For this review, use the dimensioned drawing (mm, ordinates from the lowest corner) and the shaded views. Give positions to 0.01 mm unless a question says otherwise; leave off trailing zeros. Write each loop counter-clockwise with the first axis right and the second up, starting at its lowest first coordinate (ties: lowest second). Pieces come first, ordered by that corner, then holes. Notation, with made-up numbers: (-34, 7.5) -> (-9, 7.5) arc R26 cw to (-9, 42.5) -> close; hole circle Ø4 at (5.25, -9). An arc over 180 degrees is marked (long way). Answer as CSV lines item,"result".
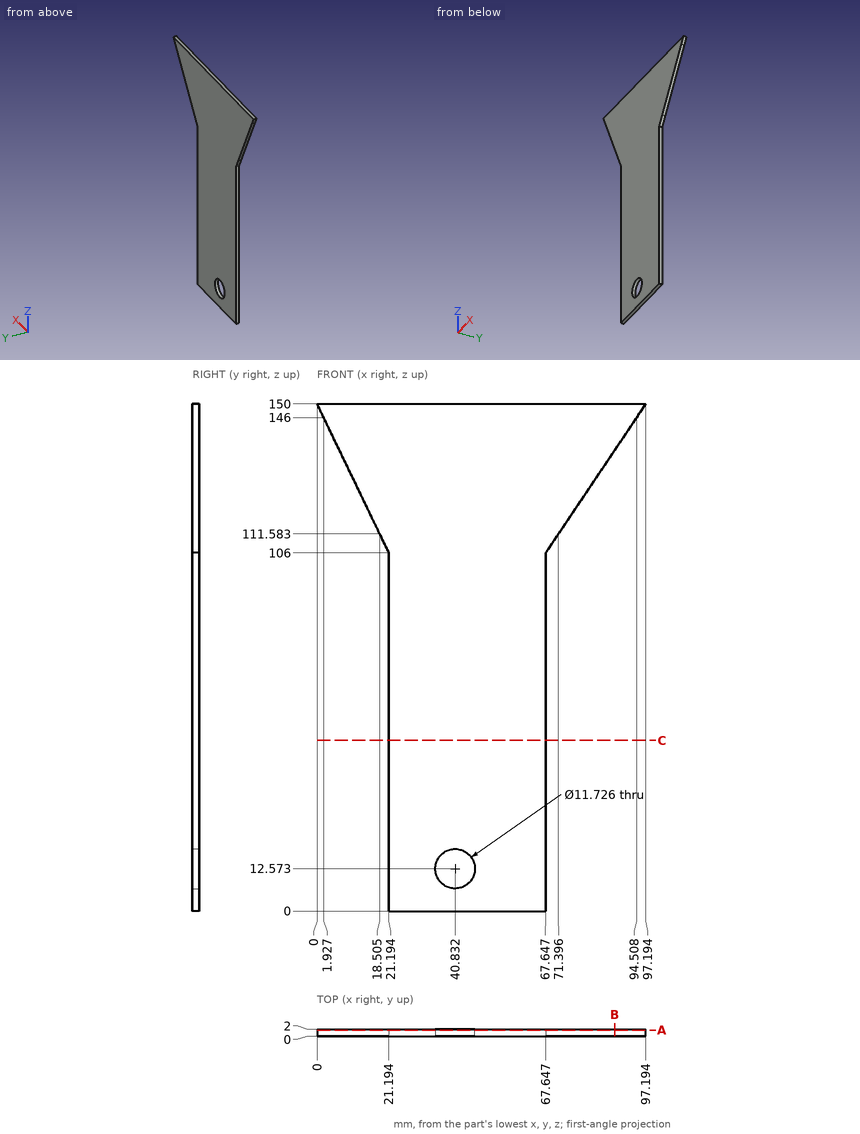
Q1. Add section B-B (x = 88). Write out the cut boundary in (y, z).
Answer block:
outline,"(0, 136.31) -> (2, 136.31) -> (2, 150) -> (0, 150) -> close"
Q2. To check wall thickness, follow probe 1 along X at (y, z) = (0.55, 101.5); probe 2 along X at (y, z) = (0.8, 13) (1 decimal); probe 3 along Z at (x, y) = (37, 1.2) (1 decimal). State the ranges of each line that lie inside material, in increasing order. Write a range as [from, to].
Answer block:
probe 1,"x = [21.19, 67.65]"
probe 2,"x = [21.2, 35], [46.7, 67.6]"
probe 3,"z = [0, 8.1], [17, 150]"
Q3. Add section A-A (y = 1.7). Write out the cut boundary in (x, z) (1 decimal).
Answer block:
outline,"(0, 150) -> (21.2, 106) -> (21.2, 0) -> (67.6, 0) -> (67.6, 106) -> (97.2, 150) -> close; hole circle Ø11.7 at (40.8, 12.6)"
Q4. Clearance check with flat-ended pins moving along their axes: pin 1 (0.6 mm diameter, centred on y = 0.5, z = 52, fed in from +X); pin 2 (0.6 mm diameter, centred on y = 1, z = 76.5, fed in from -X). State where each tip first meets the part, or that it passes through.
Answer block:
pin 1,"stops at x = 67.65"
pin 2,"stops at x = 21.19"
Q5. Add section C-C (z = 50.5). Write out the cut boundary in (x, y).
Answer block:
outline,"(21.19, 0) -> (67.65, 0) -> (67.65, 2) -> (21.19, 2) -> close"
